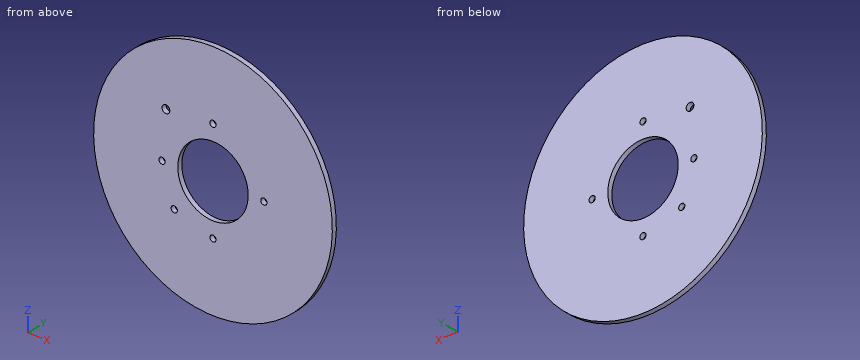
from build123d import *

# Parameters (mm, degrees)
SKETCH1_R           = 77.4600051
BOSS_EXTRUDE1_DEPTH = 3.175
SKETCH20_R          = 22.86
SKETCH20_R_2        = 2.0193
CUT_EXTRUDE10_DEPTH = 251.865681086
SKETCH21_R          = 2.0193
CUT_EXTRUDE11_DEPTH = 251.865681086
SKETCH23_R          = 2.54
CUT_EXTRUDE13_DEPTH = 3.175


with BuildPart() as part:
    # Sketch1 → Boss-Extrude1 (new body)
    with BuildSketch(Plane(origin=(0, 0, 0), x_dir=(1, 0, 0), z_dir=(0, 1, 0))):
        with Locations(Location((0, 0, 0), (0, 0, 270))):
            Circle(SKETCH1_R)
    extrude(amount=BOSS_EXTRUDE1_DEPTH)

    # Sketch20 → Cut-Extrude10 (cut, through all)
    with BuildSketch(Plane(origin=(-73.768816189, 25.4, -121.080352405), x_dir=(1, 0, 0), z_dir=(0, 1, 0))):
        with Locations(Location((73.768816189, -121.080352405, 0), (0, 0, 270))):
            Circle(SKETCH20_R)
        with Locations(Location((73.768816189, -88.060352405, 0), (0, 0, 270))):
            Circle(SKETCH20_R_2)
        with Locations(Location((106.788816189, -121.080352405, 0), (0, 0, 270))):
            Circle(SKETCH20_R_2)
        with Locations(Location((73.768816189, -154.100352405, 0), (0, 0, 270))):
            Circle(SKETCH20_R_2)
        with Locations(Location((40.748816189, -121.080352405, 0), (0, 0, 270))):
            Circle(SKETCH20_R_2)
    extrude(amount=-CUT_EXTRUDE10_DEPTH, mode=Mode.SUBTRACT)

    # Sketch21 → Cut-Extrude11 (cut, through all)
    with BuildSketch(Plane(origin=(-73.768816189, 25.4, -121.080352405), x_dir=(1, 0, 0), z_dir=(0, 1, 0))):
        with Locations(Location((48.605023435, -95.916559651, 0), (0, 0, 270))):
            Circle(SKETCH21_R)
    extrude(amount=-CUT_EXTRUDE11_DEPTH, mode=Mode.SUBTRACT)

    # Sketch23 → Cut-Extrude13 (cut)
    with BuildSketch(Plane(origin=(-73.768816189, 0, -121.080352405), x_dir=(1, 0, 0), z_dir=(0, -1, 0))):
        with Locations(Location((43.216869762, 151.632298832, 0), (0, 0, 270))):
            Circle(SKETCH23_R)
    extrude(amount=-CUT_EXTRUDE13_DEPTH, mode=Mode.SUBTRACT)


solid = part.part
Design review of the part built by this model. Coordinates are the model's own, in mm. Give positions to 0.01 mm unless a question says otherwise; leave off trailing zeros. Loops run counter-clockwise (first coordinate to the right, second up) from the corner with the lowest first, then second, coordinate; pieces in that order, holes last. Notation, with made-up numbers: (-5.75, -28.5) - (1.25, -28.5) arc R28 cw to (1.25, -3.5) - close; hole circle Ø1 at (-27.5, 42.25). An arc over 180 degrees is marked (long way). Use CSV: the item, a comma, the result in double quotes. Start each with the question number.
1. Add section C-C (z = -33.02). State the section outline as (x, y) points (3 decimals).
2. Add section A-A (z = 0). State the section outline as (x, y) points (3 decimals).
3. Add section D-D (y = 2.2). State the section outline as (x, z) points.
4. Add section B-B (x = 33.02). State the section outline as (y, z) points (3 decimals).
5. Wall thickness on L1, parallel to X at y = 1.2, z = 0; L2, parallel to Z at x = 1, y = 0.4; L3, parallel to Z at x = -19, y = 2.75: over which ranges is each line inside the solid? List them lowest first.
6. Insertion check: P1, Ø3.5, axis at x = 0, z = 33.02, coming from the -Y side. The pin has a flat end and moves straight along its axis. Give the tip position at first contact, or say it passes through.
Results found:
1,outline,"(-70.069, 0) - (-2.019, 0) - (-2.019, 3.175) - (-70.069, 3.175) - close; (2.019, 0) - (70.069, 0) - (70.069, 3.175) - (2.019, 3.175) - close"
2,outline,"(-77.46, 0) - (-35.039, 0) - (-35.039, 3.175) - (-77.46, 3.175) - close; (-31.001, 0) - (-22.86, 0) - (-22.86, 3.175) - (-31.001, 3.175) - close; (22.86, 0) - (31.001, 0) - (31.001, 3.175) - (22.86, 3.175) - close; (35.039, 0) - (77.46, 0) - (77.46, 3.175) - (35.039, 3.175) - close"
3,outline,"circle Ø154.92 at (0, 0); hole circle Ø4.04 at (-33.02, 0); hole circle Ø5.08 at (-30.55, 30.55); hole circle Ø4.04 at (-25.16, -25.16); hole circle Ø45.72 at (0, 0); hole circle Ø4.04 at (0, -33.02); hole circle Ø4.04 at (0, 33.02); hole circle Ø4.04 at (33.02, 0)"
4,outline,"(0, -70.069) - (3.175, -70.069) - (3.175, -2.019) - (0, -2.019) - close; (0, 2.019) - (3.175, 2.019) - (3.175, 70.069) - (0, 70.069) - close"
5,L1,"x = -77.46 to -35.04, -31 to -22.86, 22.86 to 31, 35.04 to 77.46"
5,L2,"z = -77.45 to -34.77, -31.27 to -22.84, 22.84 to 31.27, 34.77 to 77.45"
5,L3,"z = -75.09 to -12.71, 12.71 to 75.09"
6,P1,"passes through"
